Build history of the part. All positions in model axes, mm. A direction names the side the tool comes from. Coordinates: 2 decimals unless noted, no trailing zeros. Order: outer loops, then holes, each group sorted by start corner. A loop starts at its lowest first (then second) coordinate and runs counter-clockwise, first axis right, second up. Notation, with made-up numbers: M -26.5,-32 L 23.5,-32 A19 ccw 23.5,-22 Z; hole C 61,60 d6. An arc over 180 degrees is marked long. Write item = value, one per line. Start each with the question number.
Q1. Pull direction Y, two halves, no side cores. Call faces 1 (the face through (-22.34, 3.82, 50)), 2 (the face through (-0.3, 5.3, 2.5)), 3 (the face through (23.846, 7.509, 24.65)): released by +Y, released by -Y, zero draft, split by the parting line, or undercut.
Q2. Band-saw the part on C-C on y = 16. Write the cut outline in (x, z).
Q3. Pin check, flat tips, straight feed: P1, Ø5, axis at x = -17.5, y = 5, coming from the +Z side; P2, Ø3, axis at y = -12, z = 37, coming from the +X side; P3, Ø1.5, axis at x = 15, z = 42.5, coming from the +Y side. Stop position of each tip, or through.
Q4. Drill centre lines: probe 1 along Y at (x, z) = (0, 1.35); probe 2 along Y at (x, z) = (0, 19.5); probe 3 along Z at (x, y) = (13.5, -3). Where is each one in solid material? Low to high.
Q5. Band-saw the part on D-D on z = 43.5. Write the cut outline in (x, y), plus the area to 3 significant figures.
Q6. Band-saw the part on A-A on x = 0. Write the cut outline in (y, z).
Q7. 3-axis set-ups, long thin cutter, end or side, ignore diameter. For faces 4 (the face through (10.382, -19.961, 25.918)), 5 (the face through (1.08, -4.88, 1.23)): which of +Z, -Z, +X, -X, +Y, -Y reach the whole face in a straight line?
```python
from build123d import *

# Parameters (mm, degrees)
F0_R     = 25
F1_DEPTH = 50
F2_T     = -2.5
F4_D     = 10
F6_D     = 15


with BuildPart() as f1:
    # F0 (on Top) → F1 (new body)
    with BuildSketch(Plane.XY):
        Circle(F0_R)
    extrude(amount=F1_DEPTH)

    # F2
    f2_openings = [f1.faces().sort_by_distance(p)[0] for p in [
        (0, 0, 50),
    ]]
    offset(amount=F2_T, openings=f2_openings)

    # F4 (through all)
    with Locations(Plane.XY.offset(2.5)):
        with Locations((0, 0)):
            Hole(F4_D / 2)

    # F6 (through all)
    with Locations(Plane.XY.offset(2.5)):
        with Locations((9.350582, -11.090602)):
            Hole(F6_D / 2)


solid = f1.part
```
Recorded:
q1.face_1 = zero draft
q1.face_2 = undercut
q1.face_3 = split by the parting line
q2.outline = M -19.21,0 L 19.21,0 L 19.21,50 L 15.82,50 L 15.82,2.5 L -15.82,2.5 L -15.82,50 L -19.21,50 Z
q3.P1 = 2.5
q3.P2 = 22.69
q3.P3 = 20.54
q4.probe_1 = -25 to -5, 5 to 25
q4.probe_2 = -25 to -22.5, 22.5 to 25
q4.probe_3 = 0 to 2.5
q5.outline = C 0,0 d50; hole C 0,0 d45
q5.area = 373 mm2
q6.outline = M -25,0 L -5,0 L -5,2.5 L -22.5,2.5 L -22.5,50 L -25,50 Z; M 5,0 L 25,0 L 25,50 L 22.5,50 L 22.5,2.5 L 5,2.5 Z
q7.face_4 = +Z
q7.face_5 = +Z, -Z
